Geometry: final body of the model. Coordinates: model frame, mm. A direction names the side the tool comes from. Give positions to 0.01 mm unless a question says otherwise; leave off trailing zeros. Write each loop counter-clockwise with the first axis right and the second up, starting at its lowest first coordinate (ties: lowest second). Pieces come first, ordered by that corner, then holes.
Q1. Section D-D (y = 0). Return the cut outline in (x, z) (3 decimals), plus the area to 3 significant figures.
Q2. Line query: line 1 (Y direction, x = -15.5, z = -38.3); line 2 (Y direction, x = 15.5, z = -32.2); line 3 (X direction, y = 15.5, z = -34.2). Output: solid intervals per line, ascending.
Q3. Section A-A (x = -15.5). Return the cut outline in (y, z) (3 decimals), plus the area to 3 significant figures.
Q4. Section C-C (z = -37.25). Return the cut outline in (x, y).
Q5. Pin query (flat end, axial travel): pin 1 Ø4 at (x, z) = (19.5, -32.5) entering from -Y; pin 2 Ø5.5 at (x, y) = (15.5, -15.5) entering from -Z (3 decimals); pin 3 Ø1 at (x, z) = (18, -33) entering from +Y. Return the tip coordinate at first contact, or that it passes through.
Q6. Mould query, pull axis X, two halves, no side actions, for faces 1 (the flat face through (-21, 0, -35)), 2 (the flat face through (3.44, 3.44, -37.925)), 3 (the flat face through (0, 21, -35)). Classes: +X half, -X half, draft (parallel to the pull), parting line (faces both ways), or undercut.
Q7. Reachability of faces 4 (the flat face through (12, 0, -33)), 5 (the cylindrical face through (17.14, 12.93, -37.95)), 6 (the flat face through (2, -5, -39.925)) from +Z, -Z, +X, -X, +Y, -Y: full face, straight path, thin tool, end or side. Return the list, or none.
from build123d import *

# Parameters (mm, degrees)
SKETCH006_R             = 4.7
PAD003_DEPTH            = 9.5
SKETCH007_W             = 12.9999948434
SKETCH007_H             = 16
POCKET002_DEPTH         = 6
SKETCH008_R             = 8
POCKET003_DEPTH         = 7.5
SKETCH009_R             = 1.65
POCKET004_DEPTH         = 9.501
SKETCH010_R             = 3.05
POCKET005_DEPTH         = 3.5
FILLET_R                = 0.4
CHAMFER001_SIZE         = 0.5
BODY002_PLACEMENT_ANGLE = 180


with BuildPart() as part:
    # Sketch006 → Pad003 (new body)
    with BuildSketch(Plane.XY):
        Polygon((-21.0000051566, 17.1500051566), (-21.0000051566, -17.1500051566), (-17.1500154699, -21.0000051566), (17.1500154699, -21.0000051566), (20.9999948434, -17.1499948434), (20.9999948434, -8), (24.9999948434, -8), (24.9999948434, 8), (20.9999948434, 8), (20.9999948434, 17.1499948434), (17.1500051566, 20.9999948434), (-17.1500051566, 20.9999948434), align=None)
        Circle(SKETCH006_R, mode=Mode.SUBTRACT)
    extrude(amount=PAD003_DEPTH)

    # Sketch007 → Pocket002 (cut)
    with BuildSketch(Plane.XY):
        with Locations((18.4999974217, 0)):
            Rectangle(SKETCH007_W, SKETCH007_H)
    extrude(amount=POCKET002_DEPTH, mode=Mode.SUBTRACT)

    # Sketch008 → Pocket003 (cut)
    with BuildSketch(Plane.XY):
        Circle(SKETCH008_R)
    extrude(amount=POCKET003_DEPTH, mode=Mode.SUBTRACT)

    # Sketch009 → Pocket004 (cut, through all)
    with BuildSketch(Plane.XY.offset(9.5)):
        with Locations((-15.5, 15.5)):
            Circle(SKETCH009_R)
        with Locations((15.5, 15.5)):
            Circle(SKETCH009_R)
        with Locations((15.5, -15.5)):
            Circle(SKETCH009_R)
        with Locations((-15.5, -15.5)):
            Circle(SKETCH009_R)
    extrude(amount=-POCKET004_DEPTH, mode=Mode.SUBTRACT)

    # Sketch010 → Pocket005 (cut)
    with BuildSketch(Plane.XY.offset(9.5)):
        with Locations((-15.5, 15.5)):
            Circle(SKETCH010_R)
        with Locations((15.5, 15.5)):
            Circle(SKETCH010_R)
        with Locations((15.5, -15.5)):
            Circle(SKETCH010_R)
        with Locations((-15.5, -15.5)):
            Circle(SKETCH010_R)
    extrude(amount=-POCKET005_DEPTH, mode=Mode.SUBTRACT)

    # Fillet
    fillet_edges = [part.edges().sort_by_distance(p)[0] for p in [
        (-4.7, 0, 9.5),
        (0, -21.000005, 9.5),
        (19.075005, -19.075, 9.5),
        (20.999995, -12.574997, 9.5),
        (22.999995, -8, 9.5),
        (24.999995, -8, 7.75),
        (24.999995, 8, 7.75),
        (22.999995, 8, 9.5),
        (20.999995, 12.574997, 9.5),
        (19.075, 19.074995, 9.5),
        (0, 20.999995, 9.5),
        (-19.075005, 19.075, 9.5),
        (-21.000005, 0, 9.5),
        (-19.07501, -19.075005, 9.5),
        (24.999995, 0, 9.5),
    ]]
    fillet(fillet_edges, radius=FILLET_R)

    # Chamfer001
    chamfer001_edges = [part.edges().sort_by_distance(p)[0] for p in [
        (12.45, 15.5, 9.5),
        (-18.55, 15.5, 9.5),
        (12.45, -15.5, 9.5),
        (-18.55, -15.5, 9.5),
    ]]
    chamfer(chamfer001_edges, length=CHAMFER001_SIZE)


with BuildPart() as part_1:
    # Body002 placement: moved
    add(part.part.moved(Location((0, 0, -30.425))).rotate(Axis((0, 0, -30.425), (1, 0, 0)), BODY002_PLACEMENT_ANGLE))


solid = part_1.part
Computed:
1. outline: (-21, -39.525) arc R0.4 ccw to (-20.6, -39.925) - (-5.1, -39.925) arc R0.4 ccw to (-4.7, -39.525) - (-4.7, -37.925) - (-8, -37.925) - (-8, -30.425) - (-21, -30.425) - close; (4.7, -39.525) arc R0.4 ccw to (5.1, -39.925) - (24.6, -39.925) arc R0.4 ccw to (25, -39.525) - (25, -36.425) - (12, -36.425) - (12, -30.425) - (8, -30.425) - (8, -37.925) - (4.7, -37.925) - close
1. area: 220 mm2
2. line 1: y = -21 to -18.55, -12.45 to 12.45, 18.55 to 21
2. line 2: y = -21 to -17.15, -13.85 to -8, 8 to 13.85, 17.15 to 21
2. line 3: x = -21 to -17.15, -13.85 to 13.85, 17.15 to 21
3. outline: (-21, -39.525) arc R0.4 ccw to (-20.6, -39.925) - (-19.05, -39.925) - (-18.55, -39.425) - (-18.55, -36.425) - (-17.15, -36.425) - (-17.15, -30.425) - (-21, -30.425) - close; (-13.85, -36.425) - (-12.45, -36.425) - (-12.45, -39.425) - (-11.95, -39.925) - (11.95, -39.925) - (12.45, -39.425) - (12.45, -36.425) - (13.85, -36.425) - (13.85, -30.425) - (-13.85, -30.425) - close; (17.15, -36.425) - (18.55, -36.425) - (18.55, -39.425) - (19.05, -39.925) - (20.6, -39.925) arc R0.4 ccw to (21, -39.525) - (21, -30.425) - (17.15, -30.425) - close
3. area: 316 mm2
4. outline: (-21, -17.15) - (-17.15, -21) - (17.15, -21) - (21, -17.15) - (21, -8) - (24.6, -8) arc R0.4 ccw to (25, -7.6) - (25, 7.6) arc R0.4 ccw to (24.6, 8) - (21, 8) - (21, 17.15) - (17.15, 21) - (-17.15, 21) - (-21, 17.15) - close; hole circle Ø6.1 at (-15.5, -15.5); hole circle Ø6.1 at (-15.5, 15.5); hole circle Ø16 at (0, 0); hole circle Ø6.1 at (15.5, -15.5); hole circle Ø6.1 at (15.5, 15.5)
5. pin 1: stops at y = -20.65
5. pin 2: stops at z = -36.425
5. pin 3: stops at y = 20.65
6. face 1: -X half
6. face 2: undercut
6. face 3: draft
7. face 4: +Z, +X
7. face 5: -Z
7. face 6: -Z, +X, -X, +Y, -Y
